from build123d import *

# Parameters (mm, degrees)
SKETCH1_R                = 20
SKETCH2_R                = 30
SKETCH3_R                = 10
CUT_EXTRUDE1_DEPTH       = 59.30951912
BOSS_EXTRUDE1_DEPTH      = 20
SKETCH7_R                = 30
SKETCH7_R_2              = 15
BOSS_EXTRUDE2_DEPTH      = 10
BOSS_EXTRUDE2_DEPTH_BACK = 70
RIB1_REACH               = 152.734
SKETCH11_WALL_W          = 352.358184706
SKETCH11_WALL_H          = 10


with BuildPart() as part:
    # Sketch1 → Loft1 section 0
    with BuildSketch(Plane(origin=(0, 0, 0), x_dir=(1, 0, 0), z_dir=(0, 1, 0))):
        Circle(SKETCH1_R)
    # Sketch2 → Loft1 section 1
    with BuildSketch(Plane(origin=(0, -40, 0), x_dir=(1, 0, 0), z_dir=(0, 1, 0))):
        Circle(SKETCH2_R)
    loft()

    # Sketch3 → Cut-Extrude1 (cut, through all)
    with BuildSketch(Plane(origin=(0, 0, 0), x_dir=(1, 0, 0), z_dir=(0, 1, 0))):
        with Locations(Location((0, 0, 0), (0, 0, 270))):
            Circle(SKETCH3_R)
    extrude(amount=-CUT_EXTRUDE1_DEPTH, mode=Mode.SUBTRACT)

    # Sketch6 → Boss-Extrude1 (add)
    with BuildSketch(Plane(origin=(0, -40, 0), x_dir=(1, 0, 0), z_dir=(0, 1, 0))):
        with BuildLine():
            ThreePointArc((-30, 0), (0, 30), (30, 0))
            Line((30, 0), (30, -40))
            Line((30, -40), (-30, -40))
            Line((-30, -40), (-30, 0))
        make_face()
    extrude(amount=-BOSS_EXTRUDE1_DEPTH)

    # Sketch7 → Boss-Extrude2 (add, two sides)
    with BuildSketch(Plane(origin=(30, 0, 0), x_dir=(0, 0, -1), z_dir=(1, 0, 0))) as boss_extrude2_sk:
        with Locations((-40, -97.360679775)):
            Circle(SKETCH7_R)
        with Locations((-40, -97.360679775)):
            Circle(SKETCH7_R_2, mode=Mode.SUBTRACT)
        with BuildLine():
            Line((-20, -75), (-20, -60))
            Line((-20, -60), (-40, -60))
            Line((-40, -60), (-40, -67.360679775))
            ThreePointArc((-40, -67.360679775), (-29.295337307, -69.335509006), (-20, -75))
        make_face()
    extrude(amount=BOSS_EXTRUDE2_DEPTH)
    extrude(boss_extrude2_sk.sketch, amount=-BOSS_EXTRUDE2_DEPTH_BACK)

    # Sketch11 wall → Rib1 (add, up to next)
    with BuildSketch(Plane(origin=(0, -60.835244504, 52.784931695), x_dir=(0, -0.85232878253, 0.52300635414), z_dir=(0, -0.52300635414, -0.85232878253)), mode=Mode.PRIVATE) as rib1_sk1:
        Rectangle(SKETCH11_WALL_W, SKETCH11_WALL_H)
    rib1_tool1 = extrude(rib1_sk1.sketch, amount=RIB1_REACH, mode=Mode.PRIVATE) - part.part
    add(rib1_tool1.solids().sort_by_distance((0, -60.835244504, 52.784931695))[0])


solid = part.part
The model under review builds one solid part; all positions refer to its coordinate system, in mm. A direction names the side the tool comes from. Give positions to 0.01 mm unless a question says otherwise; leave off trailing zeros. Loops run counter-clockwise (first coordinate to the right, second up) from the corner with the lowest first, then second, coordinate; pieces in that order, holes last. Notation, with made-up numbers: (32, -9.5) -> (72, -9.5) arc R20 cw to (72, -3.5) -> close; hole circle Ø11 at (19, 59). An arc over 180 degrees is marked (long way). Answer as a JSON object with one key per item and string values. Group by question number.
Q1. Insertion check: pin 1 (13 mm diameter, centred on y = -62.5, z = 59, fed in from -X); pin 2 (8 mm diameter, centred on x = 27, y = -57.5, fed in from +Z); pin 3 (8 mm diameter, centred on x = 37, z = 33, fed in from +Y); pin 4 (24 mm diameter, centred on y = -97.36, z = 40, fed in from +X). Each pin has a flat end and moves straight along its axis. Give the tip position at first contact, or say it passes through.
Q2. Tool access review of faces 4 (the flat face through (5, -58, 46)), 5 (the flat face through (-30, -50, 20)), 6 (the flat face through (30, -50, 20)): name each direction out of +Z, -Z, +X, -X, +Y, -Y from which nothing blocks a thin tool from reaching the whole face with its end or side.
Q3. Wall thickness on line 1 along Z through (x, y) = (-3, -20); line 2 along Z through (x, y) = (3, -37); line 3 along Y through (x, z) = (-5.5, 50): over which ranges is each line inside the solid? List them lowest first.
Q4. Take a section at B-B (z = 48). Write out the cut boundary in (x, y), plus the area to 3 significant figures.
Q5. Take a section at D-D (y = -25). Write out the cut boundary in (x, z).
Q6. Draft analysis for pull direction Z (two halves, no side actions). For faces 1 (the flat face through (35, -60, 30)), 2 (the conical face through (-5.19, -15.84, 23.39)), 3 (the cylindrical face through (-9.76, -19.72, -2.17)), state which applies: pulls with the +Z half, pulls with the -Z half, needs draft (parallel to the pull), parting line crosses it, or undercut.
Q7. Take a section at A-A (y = -95). Write out the cut boundary in (x, z).
Q8. Take a section at C-C (x = 0). Write out the cut boundary in (y, z).
Answer below:
{
 "1": {"pin 1": "stops at x = -5", "pin 2": "stops at z = 40", "pin 3": "stops at y = -60", "pin 4": "passes through"},
 "2": {"face 4": "+Z, +X, +Y", "face 5": "+Z, -Z, -X, +Y", "face 6": "+Z, -Z, +X, +Y"},
 "3": {"line 1": "z = -24.82 to -9.54, 9.54 to 24.82", "line 2": "z = -29.1 to -9.54, 9.54 to 29.1", "line 3": "y = -125.64 to -108.54, -86.18 to -69.08"},
 "4": {"outline": "(-40, -126.27) -> (40, -126.27) -> (40, -110.05) -> (-40, -110.05) -> close; (-40, -84.67) -> (40, -84.67) -> (40, -68.45) -> (5, -68.45) -> (5, -53.04) -> (-5, -53.04) -> (-5, -68.45) -> (-40, -68.45) -> close", "area": "2,750 mm2"},
 "5": {"outline": "circle Ø52.5 at (0, 0); hole circle Ø20 at (0, 0)"},
 "6": {"face 1": "needs draft", "face 2": "parting line crosses it", "face 3": "undercut"},
 "7": {"outline": "(-40, 10.09) -> (40, 10.09) -> (40, 25.19) -> (-40, 25.19) -> close; (-40, 54.81) -> (40, 54.81) -> (40, 69.91) -> (-40, 69.91) -> close"},
 "8": {"outline": "(-81.67, 65.57) arc R30 ccw (long way) to (-75, 20) -> (-60, 20) -> (-60, -30) -> (-40, -30) -> (0, -20) -> (0, -10) -> (-40, -10) -> (-40, 10) -> (0, 10) -> (0, 20) -> (-40, 30) -> (-40, 40) -> close; hole circle Ø30 at (-97.36, 40)"}
}
